Work out the finished part from the listing and answer in its coordinate system (mm). Face numbers are marked on the shaded views. Give positions to 0.01 mm unless a question says otherwise; leave off trailing zeros. Order: outer loops, then holes, each group sorted by start corner. A loop starts at its lowest first (then second) coordinate and runs counter-clockwise, first axis right, second up.
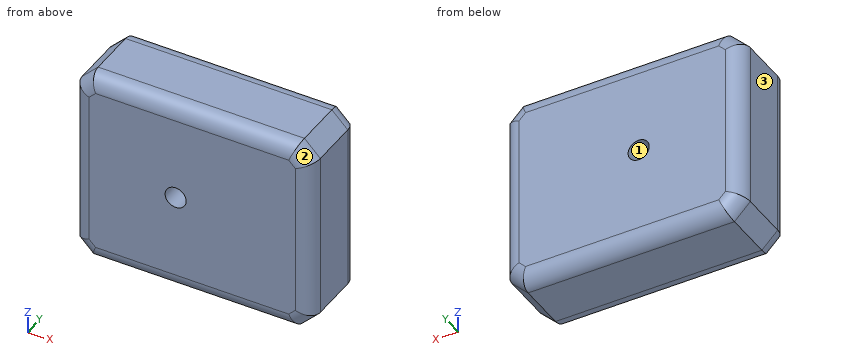
```python
from build123d import *

# Parameters (mm, degrees)
F0_W     = 76.2
F0_H     = 63.5
F1_DEPTH = 25.4
F2_SIZE  = 5.08
F3_R     = 5.08
F5_D     = 6.7564


with BuildPart() as f1:
    # F0 (on Front) → F1 (new body)
    with BuildSketch(Plane.XZ):
        with Locations((38.1, 31.75)):
            Rectangle(F0_W, F0_H)
    extrude(amount=F1_DEPTH)

    # F2
    f2_edges = [f1.edges().sort_by_distance(p)[0] for p in [
        (0, -12.7, 63.5),
        (76.2, -12.7, 63.5),
        (76.2, -12.7, 0),
        (0, -12.7, 0),
    ]]
    chamfer(f2_edges, length=F2_SIZE)

    # F3
    f3_edges = [f1.edges().sort_by_distance(p)[0] for p in [
        (0, -25.4, 31.75),
        (2.54, -25.4, 60.96),
        (38.1, -25.4, 63.5),
        (73.66, -25.4, 60.96),
        (76.2, -25.4, 31.75),
        (73.66, -25.4, 2.54),
        (38.1, -25.4, 0),
        (2.54, -25.4, 2.54),
        (38.1, 0, 0),
        (2.54, 0, 2.54),
        (0, 0, 31.75),
        (2.54, 0, 60.96),
        (38.1, 0, 63.5),
        (73.66, 0, 60.96),
        (73.66, 0, 2.54),
        (76.2, 0, 31.75),
    ]]
    fillet(f3_edges, radius=F3_R)

    # F5 (through all)
    with Locations(Plane.XZ.offset(25.4)):
        with Locations((32.8130275011, 31.9233834743)):
            Hole(F5_D / 2)


solid = f1.part
```
1. Straight lines are drawn through the part: probe 1 along Y at (x, z) = (65.5, 58.5); probe 2 along X at (y, z) = (-6.75, 32); probe 3 along Z at (x, y) = (33.5, -16.75). For each, find the intervals that lie inside material, in ascending order.
Findings below:
probe 1: y = -25.4 to 0
probe 2: x = 0 to 29.44, 36.19 to 76.2
probe 3: z = 0 to 28.62, 35.23 to 63.5
2. Given P1, Ø5.5, axis at x = 32.81, z = 31.92, coming from the +Y side, flat-ended and moving along its own axis, determine where the tip first touches the part or whether it passes through.
Findings below:
P1: passes through
3. The part is cut by section A-A (y = -2). Write down the section's boundary in (x, z), then the cut area to 3 significant figures.
Findings below:
outline: (1.04, 5.51) - (5.51, 1.04) - (70.69, 1.04) - (75.16, 5.51) - (75.16, 57.99) - (70.69, 62.46) - (5.51, 62.46) - (1.04, 57.99) - close; hole circle Ø6.76 at (32.81, 31.92)
area: 4,480 mm2
4. The part is cut by section B-B (y = -22). Write down the section's boundary in (x, z).
Findings below:
outline: (0.29, 5.2) - (5.2, 0.29) - (71, 0.29) - (75.91, 5.2) - (75.91, 58.3) - (71, 63.21) - (5.2, 63.21) - (0.29, 58.3) - close; hole circle Ø6.76 at (32.81, 31.92)
5. The mould has two halves that part along X. Classify the marked faces 1, 2 and 3: pulls with the +X half, pulls with the -X half, needs draft (parallel to the pull), parting line crosses it, or undercut.
Findings below:
face 1: undercut
face 2: pulls with the +X half
face 3: pulls with the -X half
